The model under review builds one solid part; all positions refer to its coordinate system, in mm. Coordinates: 2 decimals unless noted, no trailing zeros. Write each loop counter-clockwise with the first axis right and the second up, starting at its lowest first coordinate (ties: lowest second). Pieces come first, ordered by that corner, then holes. Notation, with made-up numbers: M 87,-33.5 L 108,-33.5 A11 cw 108,-20.5 Z; hole C 10,61 d4. An arc over 180 degrees is marked long. Answer as a JSON object with one key per item and string values.
```python
from build123d import *

# Parameters (mm, degrees)
F2_R     = 20
F3_DEPTH = 25
F6_R     = 67.15
F7_DEPTH = 1675


with BuildPart() as f3:
    # F2 (on offset) → F3 (new body)
    with BuildSketch(Plane.YZ.offset(-22)):
        with BuildLine():
            Line((0, 40), (-75, 40))
            Line((-75, 40), (-75, -40))
            Line((-75, -40), (0, -40))
            ThreePointArc((0, -40), (40, 0), (0, 40))
        make_face()
        Circle(F2_R, mode=Mode.SUBTRACT)
    extrude(amount=-F3_DEPTH)


with BuildPart() as f5_1:
    # F5: instance of F3
    add(f3.part.mirror(Plane.YZ))


with BuildPart() as f3_1:
    add(f3.part)

    add(f5_1.part)  # F7 merges F5_1
    # F6 (on face) → F7 (join, through all)
    with BuildSketch(Plane.XZ.offset(75)):
        Circle(F6_R)
    extrude(amount=F7_DEPTH)


solid = f3_1.part
```
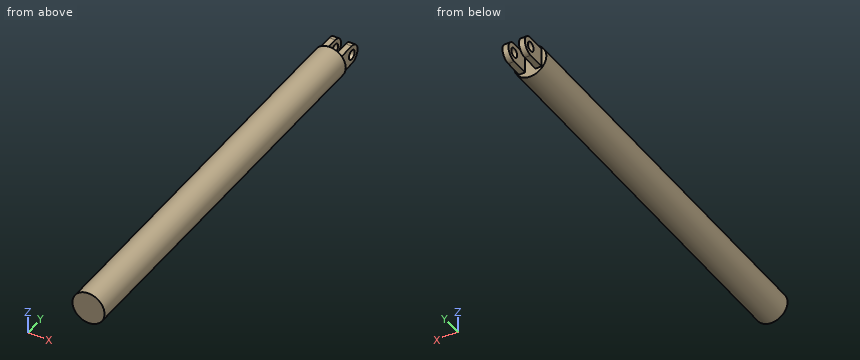
(1) Add section C-C on x = 0. Give the boundary of the cut face in (y, z), and give its area (3 significant figures).
Results list:
{"outline": "M -1750,-67.15 L -75,-67.15 L -75,67.15 L -1750,67.15 Z", "area": "225,000 mm²"}
(2) For pin 1 Ø20 at (x, y) = (-40.5, -37.5) entering from +Z; pin 2 Ø1.5 at (y, z) = (-1409, -22.5) entering from -X; pin 3 Ø6 at (y, z) = (-1034, 51) entering from +X, all flat-tipped, find the tip position at first contact; note any pin that passes through.
Results list:
{"pin 1": "z = 40", "pin 2": "x = -63.53", "pin 3": "x = 46.96"}
(3) Add section B-B on y = -117. Give the boundary of the cut face in (x, z).
Results list:
{"outline": "C 0,0 d134.3"}
(4) Add section A-A on z = 0. Give the boundary of the cut face in (x, y).
Results list:
{"outline": "M -67.15,-1750 L 67.15,-1750 L 67.15,-75 L 47,-75 L 47,-20 L 22,-20 L 22,-75 L -22,-75 L -22,-20 L -47,-20 L -47,-75 L -67.15,-75 Z; M -47,20 L -22,20 L -22,40 L -47,40 Z; M 22,20 L 47,20 L 47,40 L 22,40 Z"}
(5) Wall thickness on line 1 along X through (y, z) = (-53, 1.5); line 2 along Y through (x, z) = (-45.5, -1); line 3 along Y through (x, z) = (-50, -39.5): over which ranges is each line inside the solid? List them lowest first. Write a range as from..to.
Results list:
{"line 1": "-47..-22, 22..47", "line 2": "-1750..-19.97, 19.97..39.99", "line 3": "-1750..-75"}
